Model file for the job. Use its own axes, mm. A direction names the side the tool comes from. Round coordinates to 2 decimals unless told otherwise and drop trailing zeros. Loops run counter-clockwise (first coordinate to the right, second up) from the corner with the lowest first, then second, coordinate; pieces in that order, holes last. Notation, with made-up numbers: M 72.5,22 L 128.5,22 A19 cw 128.5,55 Z; hole C 7.25,66 d3. An arc over 180 degrees is marked long. Use a Markdown table: item, result. Add a question column.
Q1. Pin check, flat tips, straight feed: pin 1 (1.3 mm diameter, centred on x = 4, y = 0.5, fed in from +Z); pin 2 (2 mm diameter, centred on x = -5, y = 1, fed in from +Z); pin 3 (5.5 mm diameter, centred on x = 2, z = -7, fed in from -Y); pin 4 (0.8 mm diameter, centred on x = 3, y = -3.5, fed in from -Z). Stop position of each tip, or through.
Q2. Probe line 1 (Z direction, x = 5, y = -0.5); line 2 (Z direction, x = -1.25, y = -4); line 3 (X direction, y = -0.5, z = 21). List the from-to ranges inside material, lowest first. Write a range as from..to.
Q3. Tool access for faces 1 (the face through (0, -1, 30)), 2 (the face through (2.87, -0.2, 22.6)), 3 (the face through (-4, -1, 8)), 4 (the face through (0, -4, 2)): list every direction of +Z, -Z, +X, -X, +Y, -Y with a clear straight run to the whole face (end or side of a thin tool).
Q4. Mould opens along X. For faces 5 (the face through (-9.233, 0, 4)), 6 (the face through (0, -5, 16)), 7 (the face through (9.467, 0, 4)), 8 (the face through (0, -1, 5.4)) say: +X half, -X half, draft (parallel to the pull), parting line (faces both ways), or undercut.
Q5. Cut at C-C (y = 2.5). Give the cut face in (x, z), plus the area to 3 significant figures.
Q6. Cut at B-B (z = 9). Give the cut face in (x, y).
Q7. Cut at A-A (x = 1.25). Give the cut face in (y, z).
Q8. Cut at D-D (z = 20). Give the cut face in (x, y), plus the area to 3 significant figures.
from build123d import *

# Parameters (mm, degrees)
SKETCH_1_W           = 22.333333334
SKETCH_1_H           = 10
EXTRUDE_1_DEPTH      = 30
SKETCH_4_W           = 1.083333334
SKETCH_4_H           = 30
CUT_EXTRUDE_1_DEPTH  = 30
SKETCH_3_R           = 2.25
CUT_EXTRUDE_2_DEPTH  = 15
SKETCH_5_OUTSIDE_W   = 30.87
SKETCH_5_OUTSIDE_H   = 19.62
SKETCH_5_OUTSIDE_W_2 = 18.7
SKETCH_5_OUTSIDE_H_2 = 8.315719237
CUT_EXTRUDE_3_DEPTH  = 30
SKETCH_10_W          = 18.7
SKETCH_10_H          = 8.304405234
EXTRUDE_2_DEPTH      = 18
SKETCH_11_W          = 20
SKETCH_11_H          = 2.687046706
CUT_EXTRUDE_5_DEPTH  = 36.702801011
CUT_EXTRUDE_6_DEPTH  = 32.955789688
SKETCH_13_W          = 18.7
SKETCH_13_H          = 5
EXTRUDE_3_DEPTH      = 5.617358528
SKETCH_14_W          = 8
SKETCH_14_H          = 5
CUT_EXTRUDE_7_DEPTH  = 33.535840608


with BuildPart() as part:
    # 草图1 → 凸台-拉伸1 (new body)
    with BuildSketch(Plane.XY):
        Rectangle(SKETCH_1_W, SKETCH_1_H)
    extrude(amount=EXTRUDE_1_DEPTH)

    # 草图4 → 切除-拉伸1 (cut)
    with BuildSketch(Plane.XZ.offset(5)):
        with Locations((-10.625, 15)):
            Rectangle(SKETCH_4_W, SKETCH_4_H)
    extrude(amount=-CUT_EXTRUDE_1_DEPTH, mode=Mode.SUBTRACT)

    # 草图3 → 切除-拉伸2 (cut)
    with BuildSketch(Plane.XY.offset(30)):
        with Locations((-4.883333333, -0.3)):
            Circle(SKETCH_3_R)
        with Locations((5.116666667, -0.3)):
            Circle(SKETCH_3_R)
    extrude(amount=-CUT_EXTRUDE_2_DEPTH, mode=Mode.SUBTRACT)

    # 草图5 outside → 切除-拉伸3 (cut)
    with BuildSketch(Plane.XY.offset(30)):
        with Locations((0.542, 0)):
            Rectangle(SKETCH_5_OUTSIDE_W, SKETCH_5_OUTSIDE_H)
        with Locations((0.116666667, -0.853454385)):
            Rectangle(SKETCH_5_OUTSIDE_W_2, SKETCH_5_OUTSIDE_H_2, mode=Mode.SUBTRACT)
    extrude(amount=-CUT_EXTRUDE_3_DEPTH, mode=Mode.SUBTRACT)

    # 草图10 → 凸台-拉伸2 (add)
    with BuildSketch(Plane(origin=(0, 0, 0), x_dir=(-1, 0, 0), z_dir=(0, 0, -1))):
        with Locations((-0.116666667, -0.847797383)):
            Rectangle(SKETCH_10_W, SKETCH_10_H)
    extrude(amount=EXTRUDE_2_DEPTH)

    # 草图11 → 切除-拉伸5 (cut, through all)
    with BuildSketch(Plane(origin=(9.466666667, 0, 0), x_dir=(0, 0, -1), z_dir=(1, 0, 0))):
        with Locations((8, -3.656476647)):
            Rectangle(SKETCH_11_W, SKETCH_11_H)
    extrude(amount=-CUT_EXTRUDE_5_DEPTH, mode=Mode.SUBTRACT)

    # 草图12 → 切除-拉伸6 (cut, through all)
    with BuildSketch(Plane.XZ.offset(2.312953294)):
        with BuildLine():
            ThreePointArc((-2.185193673, -12.99813966), (-4.733333333, -10.45), (-7.281472993, -12.99813966))
            Line((-7.281472993, -12.99813966), (-2.185193673, -12.99813966))
        make_face()
        with BuildLine():
            Line((-2.185193673, -12.99813966), (-7.281472993, -12.99813966))
            ThreePointArc((-7.281472993, -12.99813966), (-4.733333333, -15.54627932), (-2.185193673, -12.99813966))
        make_face()
        with BuildLine():
            ThreePointArc((7.514806327, -12.99813966), (4.966666667, -10.45), (2.418527007, -12.99813966))
            Line((2.418527007, -12.99813966), (7.514806327, -12.99813966))
        make_face()
        with BuildLine():
            Line((7.514806327, -12.99813966), (2.418527007, -12.99813966))
            ThreePointArc((2.418527007, -12.99813966), (4.966666667, -15.54627932), (7.514806327, -12.99813966))
        make_face()
    extrude(amount=-CUT_EXTRUDE_6_DEPTH, mode=Mode.SUBTRACT)

    # 草图13 → 凸台-拉伸3 (add)
    with BuildSketch(Plane(origin=(0, 3.304405234, 0), x_dir=(1, 0, 0), z_dir=(0, 1, 0))):
        with Locations((0.116666667, 20.5)):
            Rectangle(SKETCH_13_W, SKETCH_13_H)
    extrude(amount=-EXTRUDE_3_DEPTH)

    # 草图14 → 切除-拉伸7 (cut, through all)
    with BuildSketch(Plane(origin=(0, 3.304405234, 0), x_dir=(1, 0, 0), z_dir=(0, 1, 0))):
        with Locations((0, -7.9)):
            Rectangle(SKETCH_14_W, SKETCH_14_H)
    extrude(amount=-CUT_EXTRUDE_7_DEPTH, mode=Mode.SUBTRACT)


solid = part.part
Checked values:
| question | item | result |
|---|---|---|
| 1 | pin 1 | stops at z = 15 |
| 1 | pin 2 | stops at z = 30 |
| 1 | pin 3 | stops at y = -2.31 |
| 1 | pin 4 | stops at z = 2 |
| 2 | line 1 | z = -23..-15.55, -10.45..15 |
| 2 | line 2 | z = 2..5.4, 10.4..30 |
| 2 | line 3 | x = -9.23..-7.12, -2.64..2.88, 7.36..9.47 |
| 3 | face 1 | +Z, +X, -X, +Y, -Y |
| 3 | face 2 | +Z |
| 3 | face 3 | +Y, -Y |
| 3 | face 4 | -Z, +X, -X, -Y |
| 4 | face 5 | -X half |
| 4 | face 6 | draft |
| 4 | face 7 | +X half |
| 4 | face 8 | undercut |
| 5 | outline | M -9.23,-23 L 9.47,-23 L 9.47,30 L -9.23,30 Z; hole C -4.73,-13 d5.1; hole M -4,5.4 L 4,5.4 L 4,10.4 L -4,10.4 Z; hole C 4.97,-13 d5.1 |
| 5 | area | 910 mm^2 |
| 6 | outline | M -9.23,-5 L -4,-5 L -4,3.3 L -9.23,3.3 Z; M 4,-5 L 9.47,-5 L 9.47,3.3 L 4,3.3 Z |
| 7 | outline | M -5,2 L -2.31,2 L -2.31,-23 L 3.3,-23 L 3.3,5.4 L -5,5.4 Z; M -5,10.4 L 3.3,10.4 L 3.3,30 L -5,30 Z |
| 8 | outline | M -9.23,-5 L 9.47,-5 L 9.47,3.3 L -9.23,3.3 Z; hole C -4.88,-0.3 d4.5; hole C 5.12,-0.3 d4.5 |
| 8 | area | 123 mm^2 |
